Part model, mm, in its own coordinate system. Face numbers are marked on the shaded views. A direction names the side the tool comes from. Coordinates: 2 decimals unless noted, no trailing zeros. Write each loop counter-clockwise with the first axis right and the second up, starting at its lowest first coordinate (ties: lowest second). Pieces come first, ordered by that corner, then holes. Notation, with made-up numbers: (27.25, -8) -> (68.25, -8) arc R14 cw to (68.25, -2) -> close; hole circle Ø1 at (45, -21). An arc over 180 degrees is marked (long way). Write item = value, one per line. Start each with the question number.
Q1. Pin check, flat tips, straight feed: P1, Ø1, axis at x = 0, z = -2.5, coming from the +Y side; P2, Ø1.5, axis at x = 2.5, z = -2.5, coming from the +Y side; P3, Ø0.9, axis at x = -3, y = 1, coming from the +Z side. Stop position of each tip, or through.
Q2. Band-saw the part on B-B, the plane y = 0.75. List the corners of the cut face in (x, z).
Q3. Band-saw the part on C-C, the plane y = 0.4. List the corners of the cut face in (x, z).
Q4. Pull direction X, two halves, no side cores. Call the marked faces 4, 5, 6 and 7: released by +X, released by -X, zero draft, split by the parting line, or undercut.
Q5. Probe line 1 (Z direction, x = -1.5, y = 1.95); line 2 (Y direction, x = 1.75, z = -4.6); line 3 (X direction, y = 0.25, z = -4.3). List the from-to ranges inside material, lowest first.
Q6. Tool access for the marked faces 1, 2 and 3: list every direction of +Z, -Z, +X, -X, +Y, -Y with a clear straight run to the whole face (end or side of a thin tool).
Q7. Band-saw the part on A-A, the plane z = -2.2. List the corners of the cut face in (x, y) (3 decimals), plus the area to 4 significant figures.
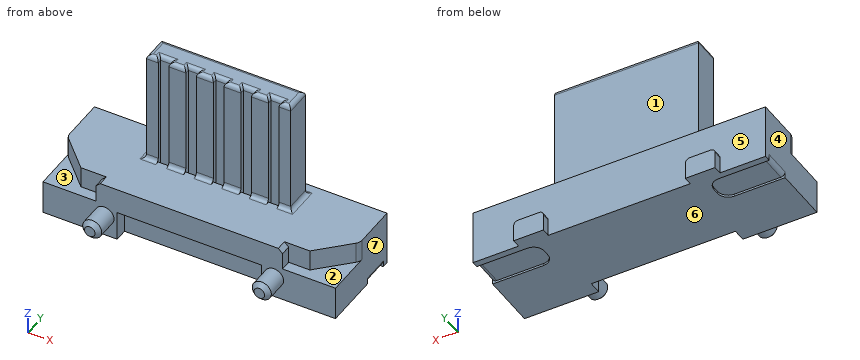
from build123d import *

# Parameters (mm, degrees)
SKETCH1_W           = 6.9
SKETCH1_H           = 1.3
BOSS_EXTRUDE1_DEPTH = 2.1
SKETCH2_W           = 3.4
SKETCH2_H           = 0.6
BOSS_EXTRUDE2_DEPTH = 2.7
SKETCH3_W           = 0.25
SKETCH3_H           = 0.1
CUT_EXTRUDE1_DEPTH  = 3
FILLET1_R           = 0.1
CUT_EXTRUDE2_DEPTH  = 0.5
FILLET3_R           = 0.2
CHAMFER1_SIZE       = 0.1
CUT_EXTRUDE3_DEPTH  = 0.05
FILLET4_R           = 0.1
SKETCH6_R           = 0.225
BOSS_EXTRUDE3_DEPTH = 0.6
CHAMFER2_SIZE       = 0.1
SKETCH7_W           = 3.4
SKETCH7_H           = 0.7
CUT_EXTRUDE4_DEPTH  = 0.3
BOSS_EXTRUDE4_DEPTH = 0.2


with BuildPart() as part:
    # Sketch1 → Boss-Extrude1 (new body)
    with BuildSketch(Plane(origin=(0, 0, 0), x_dir=(1, 0, 0), z_dir=(0, 1, 0))):
        with Locations((0, 4.15)):
            Rectangle(SKETCH1_W, SKETCH1_H)
    extrude(amount=BOSS_EXTRUDE1_DEPTH)

    # Sketch2 → Boss-Extrude2 (add)
    with BuildSketch(Plane.XY.offset(-3.5)):
        with Locations((0, 1.5)):
            Rectangle(SKETCH2_W, SKETCH2_H)
    extrude(amount=BOSS_EXTRUDE2_DEPTH)

    # Sketch3 → Cut-Extrude1 (cut)
    with BuildSketch(Plane.XY.offset(-0.8)):
        with Locations((-1.3, 1.25)):
            Rectangle(SKETCH3_W, SKETCH3_H)
        with Locations((-0.65, 1.25)):
            Rectangle(SKETCH3_W, SKETCH3_H)
        with Locations((0, 1.25)):
            Rectangle(SKETCH3_W, SKETCH3_H)
        with Locations((0.65, 1.25)):
            Rectangle(SKETCH3_W, SKETCH3_H)
        with Locations((1.3, 1.25)):
            Rectangle(SKETCH3_W, SKETCH3_H)
    extrude(amount=-CUT_EXTRUDE1_DEPTH, mode=Mode.SUBTRACT)

    # Fillet1
    fillet1_edges = [part.edges().sort_by_distance(p)[0] for p in [
        (0, 1.8, -0.8),
        (1.7, 1.5, -0.8),
        (1.5625, 1.2, -0.8),
        (-1.5625, 1.2, -0.8),
        (-1.7, 1.5, -0.8),
        (-1.7, 1.5, -3.5),
        (0, 1.8, -3.5),
        (1.7, 1.5, -3.5),
        (1.5625, 1.2, -3.5),
        (-1.5625, 1.2, -3.5),
        (0.975, 1.2, -0.8),
        (0.775, 1.25, -0.8),
        (0.65, 1.3, -0.8),
        (0.525, 1.25, -0.8),
        (0.325, 1.2, -0.8),
        (0.125, 1.25, -0.8),
        (0, 1.3, -0.8),
        (-0.125, 1.25, -0.8),
        (-0.325, 1.2, -0.8),
        (-0.525, 1.25, -0.8),
        (-0.65, 1.3, -0.8),
        (-0.775, 1.25, -0.8),
        (-0.975, 1.2, -0.8),
        (-1.175, 1.25, -0.8),
        (-1.3, 1.3, -0.8),
        (-1.425, 1.25, -0.8),
        (1.425, 1.25, -0.8),
        (1.3, 1.3, -0.8),
        (1.175, 1.25, -0.8),
        (0.975, 1.2, -3.5),
        (0.325, 1.2, -3.5),
        (-0.325, 1.2, -3.5),
        (-0.975, 1.2, -3.5),
    ]]
    fillet(fillet1_edges, radius=FILLET1_R)

    # Sketch4 → Cut-Extrude2 (cut)
    with BuildSketch(Plane.XY.offset(-3.5)):
        Polygon((-2.7, 0.25), (-3.45, 1), (-3.45, 0), (-2.2, 0), (-2.2, 0.25), align=None)
        Polygon((3.45, 1), (2.7, 0.25), (2.2, 0.25), (2.2, 0), (3.45, 0), align=None)
    extrude(amount=-CUT_EXTRUDE2_DEPTH, mode=Mode.SUBTRACT)

    # Fillet3
    fillet3_edges = [part.edges().sort_by_distance(p)[0] for p in [
        (-3.45, 1, -3.75),
        (3.45, 1, -3.75),
    ]]
    fillet(fillet3_edges, radius=FILLET3_R)

    # Chamfer1
    chamfer1_edges = [part.edges().sort_by_distance(p)[0] for p in [
        (-2.2, 0.125, -3.5),
        (2.2, 0.125, -3.5),
    ]]
    chamfer(chamfer1_edges, length=CHAMFER1_SIZE)

    # Sketch5 → Cut-Extrude3 (cut)
    with BuildSketch(Plane(origin=(0, 0, -4.8), x_dir=(-1, 0, 0), z_dir=(0, 0, -1))):
        with BuildLine():
            Line((-3.45, 1.95), (-2.25, 1.95))
            ThreePointArc((-2.25, 1.95), (-2.073223305, 1.876776695), (-2, 1.7))
            Line((-2, 1.7), (-2, 1.55))
            ThreePointArc((-2, 1.55), (-2.073223305, 1.373223305), (-2.25, 1.3))
            Line((-2.25, 1.3), (-3.45, 1.3))
            Line((-3.45, 1.3), (-3.45, 1.95))
        make_face()
        with BuildLine():
            Line((3.45, 1.95), (2.25, 1.95))
            ThreePointArc((2.25, 1.95), (2.073223305, 1.876776695), (2, 1.7))
            Line((2, 1.7), (2, 1.55))
            ThreePointArc((2, 1.55), (2.073223305, 1.373223305), (2.25, 1.3))
            Line((2.25, 1.3), (3.45, 1.3))
            Line((3.45, 1.3), (3.45, 1.95))
        make_face()
    extrude(amount=-CUT_EXTRUDE3_DEPTH, mode=Mode.SUBTRACT)

    # Fillet4
    fillet4_edges = [part.edges().sort_by_distance(p)[0] for p in [
        (3.45, 1.625, -4.75),
        (-3.45, 1.625, -4.75),
    ]]
    fillet(fillet4_edges, radius=FILLET4_R)

    # Sketch6 → Boss-Extrude3 (add)
    with BuildSketch(Plane.XZ):
        with Locations((2, -4.3)):
            Circle(SKETCH6_R)
        with Locations((-2, -4.3)):
            Circle(SKETCH6_R)
    extrude(amount=BOSS_EXTRUDE3_DEPTH)

    # Chamfer2
    chamfer2_edges = [part.edges().sort_by_distance(p)[0] for p in [
        (1.775, -0.6, -4.3),
        (-2.225, -0.6, -4.3),
    ]]
    chamfer(chamfer2_edges, length=CHAMFER2_SIZE)

    # Sketch7 → Cut-Extrude4 (cut)
    with BuildSketch(Plane.XZ):
        with Locations((0, -4.45)):
            Rectangle(SKETCH7_W, SKETCH7_H)
    extrude(amount=-CUT_EXTRUDE4_DEPTH, mode=Mode.SUBTRACT)

    # Sketch8 → Boss-Extrude4 (add)
    with BuildSketch(Plane(origin=(0, 2.1, 0), x_dir=(1, 0, 0), z_dir=(0, 1, 0))):
        with BuildLine():
            Line((-2.375, 4.8), (-1.675, 4.8))
            Line((-1.675, 4.8), (-1.675, 4.4))
            ThreePointArc((-1.675, 4.4), (-1.704289322, 4.329289322), (-1.775, 4.3))
            Line((-1.775, 4.3), (-2.275, 4.3))
            ThreePointArc((-2.275, 4.3), (-2.345710678, 4.329289322), (-2.375, 4.4))
            Line((-2.375, 4.4), (-2.375, 4.8))
        make_face()
        with BuildLine():
            Line((1.675, 4.8), (2.375, 4.8))
            Line((2.375, 4.8), (2.375, 4.4))
            ThreePointArc((2.375, 4.4), (2.345710678, 4.329289322), (2.275, 4.3))
            Line((2.275, 4.3), (1.775, 4.3))
            ThreePointArc((1.775, 4.3), (1.704289322, 4.329289322), (1.675, 4.4))
            Line((1.675, 4.4), (1.675, 4.8))
        make_face()
    extrude(amount=BOSS_EXTRUDE4_DEPTH)


solid = part.part
Ans:
q1.P1 = 1.8
q1.P2 = through
q1.P3 = -3.5
q2.outline = (-3.45, -4.8) -> (3.45, -4.8) -> (3.45, -4) -> (3.2, -4) -> (3.2, -3.5) -> (-3.2, -3.5) -> (-3.2, -4) -> (-3.45, -4) -> close
q3.outline = (-3.45, -4.8) -> (3.45, -4.8) -> (3.45, -4) -> (2.85, -4) -> (2.85, -3.5) -> (-2.85, -3.5) -> (-2.85, -4) -> (-3.45, -4) -> close
q4.face_4 = released by -X
q4.face_5 = undercut
q4.face_6 = zero draft
q4.face_7 = released by +X
q5.line_1 = -4.8 to -3.5
q5.line_2 = 0 to 2.3
q5.line_3 = -3.45 to -1.7, 1.7 to 3.45
q6.face_1 = +Z, +X, -X, +Y
q6.face_2 = +Z, +X, -Y
q6.face_3 = +Z, -X, -Y
q7.outline = (-1.7, 1.2) -> (-1.425, 1.2) -> (-1.425, 1.3) -> (-1.175, 1.3) -> (-1.175, 1.2) -> (-0.775, 1.2) -> (-0.775, 1.3) -> (-0.525, 1.3) -> (-0.525, 1.2) -> (-0.125, 1.2) -> (-0.125, 1.3) -> (0.125, 1.3) -> (0.125, 1.2) -> (0.525, 1.2) -> (0.525, 1.3) -> (0.775, 1.3) -> (0.775, 1.2) -> (1.175, 1.2) -> (1.175, 1.3) -> (1.425, 1.3) -> (1.425, 1.2) -> (1.7, 1.2) -> (1.7, 1.8) -> (-1.7, 1.8) -> close
q7.area = 1.915 mm2
